from build123d import *

# Parameters (mm, degrees)
BASE_FLANGE1_DEPTH       = 1.99898
SKETCHED_START           = -17
SKETCHED_BEND1_OUTLINE_W = 22.201670932
SKETCHED_BEND1_OUTLINE_H = 1.99898
SKETCHED_BEND1_DEPTH     = 17.02505456
SKETCHED_START_2         = 0.266062511
SKETCHED_BEND1_2_DEPTH   = 1.732917489
SKETCHED_BEND1_3_DEPTH   = 2.73558
SKETCHED_START_3         = -7.17537008
SKETCHED_BEND1_4_DEPTH   = 22.201670932
SKETCH21_W               = 1.905
SKETCH21_H               = 1.99898
SKETCH17_R               = 1.905
CUT_EXTRUDE4_DEPTH       = 2.54


with BuildPart() as part:
    # Base-Flange1: sheet metal written as solids
    # Sketch1 → Base-Flange1 (new body)
    with BuildSketch(Plane(origin=(0, 0, 0), x_dir=(1, 0, 0), z_dir=(0, 1, 0))):
        with BuildLine():
            Line((15.026300852, -4.572), (15.026300852, 4.572))
            ThreePointArc((15.026300852, 4.572), (3.925465386, 15.672835466), (-7.17537008, 4.572))
            Line((-7.17537008, 4.572), (-7.17537008, -4.572))
            ThreePointArc((-7.17537008, -4.572), (3.925465386, -15.672835466), (15.026300852, -4.572))
        make_face()
    extrude(amount=-BASE_FLANGE1_DEPTH)

    # Sketched Bend1: read off the stored shape, not the designer's step
    # Sketched Bend1 outline → Sketched Bend1 (cut)
    with BuildSketch(Plane.XY.offset(SKETCHED_START)):
        with Locations((3.925465386, -0.99949)):
            Rectangle(SKETCHED_BEND1_OUTLINE_W, SKETCHED_BEND1_OUTLINE_H)
    extrude(amount=SKETCHED_BEND1_DEPTH, mode=Mode.SUBTRACT)

    # Sketched Bend1 2 outline → Sketched Bend1 2 (add)
    with BuildSketch(Plane.XY.offset(SKETCHED_START_2)):
        with BuildLine():
            Line((15.026300852, 0), (15.026300852, 5.317136205))
            ThreePointArc((15.026300852, 5.317136205), (3.925465386, 16.417971671), (-7.17537008, 5.317136205))
            Line((-7.17537008, 5.317136205), (-7.17537008, 0))
            Line((-7.17537008, 0), (15.026300852, 0))
        make_face()
    extrude(amount=SKETCHED_BEND1_2_DEPTH)

    # Sketched Bend1 3 outline → Sketched Bend1 3 (add)
    with BuildSketch(Plane.XY):
        with BuildLine():
            Line((15.026300852, 0), (15.026300852, 5.317136205))
            ThreePointArc((15.026300852, 5.317136205), (3.925465386, 16.417971671), (-7.17537008, 5.317136205))
            Line((-7.17537008, 5.317136205), (-7.17537008, 0))
            Line((-7.17537008, 0), (15.026300852, 0))
        make_face()
    extrude(amount=SKETCHED_BEND1_3_DEPTH)

    # Sketched Bend1 4 outline → Sketched Bend1 4 (cut)
    with BuildSketch(Plane.YZ.offset(SKETCHED_START_3)):
        with BuildLine():
            ThreePointArc((0, 2.73558), (0.215745145, 2.214725145), (0.7366, 1.99898))
            Line((0.7366, 1.99898), (18, 1.99898))
            Line((18, 1.99898), (18, 2.73558))
            Line((18, 2.73558), (0, 2.73558))
        make_face()
        with BuildLine():
            Line((18, -2), (18, -1e-08))
            Line((18, -1e-08), (0.7366, 0))
            ThreePointArc((0.7366, 0), (-1.197747168, 0.801232832), (-1.99898, 2.73558))
            Line((-1.99898, 2.73558), (-1.99898, 0.02505456))
            Line((-1.99898, 0.02505456), (0, 0.02505456))
            Line((0, 0.02505456), (0, -2))
            Line((0, -2), (18, -2))
        make_face()
    extrude(amount=SKETCHED_BEND1_4_DEPTH, mode=Mode.SUBTRACT)

    # Sketch21 → Hole1 (revolve, cut)
    with BuildSketch(Plane(origin=(3.925465386, 0, 4.572), x_dir=(0, 0, 1), z_dir=(1, 0, 0))):
        with Locations((0.9525, 0.99949)):
            Rectangle(SKETCH21_W, SKETCH21_H)
    revolve(axis=Axis((3.925465386, -110, 4.572), (0, 1, 0)), mode=Mode.SUBTRACT)

    # Sketch17 → Cut-Extrude4 (cut)
    with BuildSketch(Plane.XY.offset(1.99898)):
        with Locations((3.997762003, 4.09330652)):
            Circle(SKETCH17_R)
    extrude(amount=-CUT_EXTRUDE4_DEPTH, mode=Mode.SUBTRACT)


solid = part.part
Design review of the part built by this model. Coordinates are the model's own, in mm. A direction names the side the tool comes from. Give positions to 0.01 mm unless a question says otherwise; leave off trailing zeros. Order: outer loops, then holes, each group sorted by start corner. A loop starts at its lowest first (then second) coordinate and runs counter-clockwise, first axis right, second up.
1. For pin 1 Ø8 at (y, z) = (14.5, 4) entering from -X; pin 2 Ø8 at (x, y) = (4, 14.5) entering from +Z; pin 3 Ø4 at (x, z) = (2.5, 9.5) entering from +Y, all flat-tipped, find the tip position at first contact; note any pin that passes through.
Solution:
pin 1: stops at x = -5.59
pin 2: stops at z = 2
pin 3: stops at y = 0
2. Add section C-C, the plane x = -1.5. State the section outline as (y, z) points.
Solution:
outline: (-2, 2.74) arc R2.74 ccw to (0.74, 0) - (15, 0) - (15, 2) - (0.74, 2) arc R0.74 cw to (0, 2.74) - (0, 14.26) - (-2, 14.26) - close
3. Add section D-D, the plane y = 1. State the section outline as (x, z) points, then the cut area to 3 significant figures.
Solution:
outline: (-7.18, 0) - (15.03, 0) - (15.03, 2) - (-7.18, 2) - close
area: 44.4 mm2
4. Mouldability with a two-part tool opening along X and no side actions: class faces 1 (the cylindrical face through (3.68, -0.99, 15.67)), 2 (the cylindrical face through (3.196, -1.013, 6.332)), 3 (the flat face through (4, 8, 1.999)) as +X half, -X half, draft (parallel to the pull), parting line (faces both ways), or undercut.
Solution:
face 1: parting line
face 2: undercut
face 3: draft
5. Add section A-A, the plane z = 6. State the section outline as (x, y) points.
Solution:
outline: (-7.08, -2) - (2.66, -2) - (2.66, 0) - (-7.08, 0) - close; (5.19, -2) - (14.93, -2) - (14.93, 0) - (5.19, 0) - close
6. Add section B-B, the plane y = 3. State the section outline as (x, z) points.
Solution:
outline: (-7.18, 0) - (2.44, 0) - (2.44, 2) - (-7.18, 2) - close; (5.56, 0) - (15.03, 0) - (15.03, 2) - (5.56, 2) - close
7. Tool access review of faces 4 (the flat face through (-7.175, 0.9, 1.7)), 5 (the flat face through (4, 0, 8)): name each direction out of +Z, -Z, +X, -X, +Y, -Y from which nothing blocks a thin tool from reaching the whole face with its end or side.
Solution:
face 4: +Z, -Z, -X, +Y, -Y
face 5: +Z, +X, -X, +Y
8. To check wall thickness, follow L1, parallel to Z at x = 4.25, y = 8.75; L2, parallel to Y at x = 7.75, z = 9.25; L3, parallel to X at y = -1, z = 14.25. State the ranges of each line that lie inside material, in increasing order.
Solution:
L1: z = 0 to 2
L2: y = -2 to 0
L3: x = -1.51 to 9.36
